Geometry: final body of the model. Coordinates: model frame, mm. A direction names the side the tool comes from. Coordinates: 2 decimals unless noted, no trailing zeros. Loops run counter-clockwise (first coordinate to the right, second up) from the corner with the lowest first, then second, coordinate; pieces in that order, holes last. Notation, with made-up numbers: (72, -40) - (120, -40) arc R17 cw to (120, -16) - close; hole circle Ø6 at (-32, -27). An arc over 180 degrees is marked (long way). Return JSON: item names as keys, results as strings.
from build123d import *

# Parameters (mm, degrees)
SKETCH1_R           = 8
BOSS_EXTRUDE1_DEPTH = 90
SKETCH2_R           = 10
BOSS_EXTRUDE2_DEPTH = 10
BOSS_EXTRUDE3_START = 10
SKETCH3_R           = 10
BOSS_EXTRUDE3_DEPTH = 10
SKETCH4_R           = 7.5
BOSS_EXTRUDE4_DEPTH = 15
BOSS_EXTRUDE5_START = 16
SKETCH5_R           = 7.5
BOSS_EXTRUDE5_DEPTH = 16
SKETCH6_R           = 2.5
CUT_EXTRUDE1_DEPTH  = 16
SKETCH7_R           = 4.5
CUT_EXTRUDE2_DEPTH  = 4
CUT_EXTRUDE3_DEPTH  = 16
SKETCH9_R           = 3
CUT_EXTRUDE4_DEPTH  = 117.53754762


with BuildPart() as part:
    # Sketch1 → Boss-Extrude1 (new body)
    with BuildSketch(Plane.XY):
        with Locations(Location((0, 0, 0), (0, 0, 180))):
            Circle(SKETCH1_R)
    extrude(amount=BOSS_EXTRUDE1_DEPTH)

    # Sketch2 → Boss-Extrude2 (add)
    with BuildSketch(Plane(origin=(0, 0, 0), x_dir=(-1, 0, 0), z_dir=(0, 0, -1))):
        Circle(SKETCH2_R)
    extrude(amount=BOSS_EXTRUDE2_DEPTH)

    # Sketch3 → Boss-Extrude3 (add)
    with BuildSketch(Plane.XY.offset(90).offset(BOSS_EXTRUDE3_START)):
        with Locations(Location((0, 0, 0), (0, 0, 180))):
            Circle(SKETCH3_R)
    extrude(amount=-BOSS_EXTRUDE3_DEPTH)

    # Sketch4 → Boss-Extrude4 (add)
    with BuildSketch(Plane.XY.offset(100)):
        Circle(SKETCH4_R)
    extrude(amount=BOSS_EXTRUDE4_DEPTH)

    # Sketch5 → Boss-Extrude5 (add)
    with BuildSketch(Plane(origin=(0, 0, -10), x_dir=(-1, 0, 0), z_dir=(0, 0, -1)).offset(BOSS_EXTRUDE5_START)):
        with Locations(Location((0, 0, 0), (0, 0, 180))):
            Circle(SKETCH5_R)
    extrude(amount=-BOSS_EXTRUDE5_DEPTH)

    # Sketch6 → Cut-Extrude1 (cut)
    with BuildSketch(Plane.XY.offset(115)):
        Circle(SKETCH6_R)
    extrude(amount=-CUT_EXTRUDE1_DEPTH, mode=Mode.SUBTRACT)

    # Sketch7 → Cut-Extrude2 (cut)
    with BuildSketch(Plane(origin=(0, 10, 0), x_dir=(-1, 0, 0), z_dir=(0, 1, 0))):
        with Locations(Location((0, 95, 0), (0, 0, 90))):
            Circle(SKETCH7_R)
        with Locations(Location((0, -5, 0), (0, 0, 90))):
            Circle(SKETCH7_R)
    extrude(amount=-CUT_EXTRUDE2_DEPTH, mode=Mode.SUBTRACT)

    # Sketch8 → Cut-Extrude3 (cut)
    with BuildSketch(Plane(origin=(0, 0, -26), x_dir=(-1, 0, 0), z_dir=(0, 0, -1))):
        with BuildLine():
            Line((-6, 4.5), (-6, -4.5))
            ThreePointArc((-6, -4.5), (-7.5, 0), (-6, 4.5))
        make_face()
        with BuildLine():
            Line((6, 4.5), (6, -4.5))
            ThreePointArc((6, -4.5), (7.5, 0), (6, 4.5))
        make_face()
    extrude(amount=-CUT_EXTRUDE3_DEPTH, mode=Mode.SUBTRACT)

    # Sketch9 → Cut-Extrude4 (cut, through all)
    with BuildSketch(Plane(origin=(6, 0, 0), x_dir=(0, 0, -1), z_dir=(1, 0, 0))):
        with Locations((19, 0)):
            Circle(SKETCH9_R)
    extrude(amount=-CUT_EXTRUDE4_DEPTH, mode=Mode.SUBTRACT)


solid = part.part
Item 1: Ray query, probe 1 along Z at (x, y) = (0, 7.6); probe 2 along Z at (x, y) = (0.75, -8); probe 3 along X at (y, z) = (-6, 106.5). Return the intervals inside material, ascending. Write a range as from..to.
Worked out:
{"probe 1": "-10..-9.5, -0.5..90.5, 99.5..100", "probe 2": "-10..0, 90..100", "probe 3": "-4.5..4.5"}
Item 2: Mould query, pull axis Z, two halves, no side actions, for faces 1 (the face through (0, 0, 99)), 2 (the face through (0.1, -7.5, -18.1)), 3 (the face through (1.352, 7.584, -0.708)). Classes: +Z half, -Z half, draft (parallel to the pull), parting line (faces both ways), or undercut.
Worked out:
{"face 1": "+Z half", "face 2": "draft", "face 3": "undercut"}
Item 3: Reachability of faces 4 (the face through (-7, 0, -10)), 5 (the face through (-7.493, 0.33, 107.395)), 6 (the face through (-0.1, 7.5, -18.1)), 7 (the face through (-6, 2, -16)), 8 (the face through (6, 2, -16)) from +Z, -Z, +X, -X, +Y, -Y: full face, straight path, thin tool, end or side. Return the list, or none.
Worked out:
{"face 4": "-Z", "face 5": "+Z", "face 6": "-Z, +Y", "face 7": "-Z, -X, +Y, -Y", "face 8": "-Z, +X, +Y, -Y"}
Item 4: Section query D-D, the plane z = 31. Return loops of the section in (x, y), and give its area (3 significant figures).
Worked out:
{"outline": "circle Ø16 at (0, 0)", "area": "201 mm^2"}
Item 5: Section query A-A, the plane y = 0. Return loops of the section in (x, z), and give its area (4 significant figures).
Worked out:
{"outline": "(-10, -10) - (-6, -10) - (-6, -16) - (6, -16) - (6, -10) - (10, -10) - (10, 0) - (8, 0) - (8, 90) - (10, 90) - (10, 100) - (7.5, 100) - (7.5, 115) - (2.5, 115) - (2.5, 99) - (-2.5, 99) - (-2.5, 115) - (-7.5, 115) - (-7.5, 100) - (-10, 100) - (-10, 90) - (-8, 90) - (-8, 0) - (-10, 0) - close; (-6, -26) - (6, -26) - (6, -22) - (-6, -22) - close", "area": "2,105 mm^2"}
Item 6: Section query B-B, the plane z = -19. Return loops of the section in (x, y).
Worked out:
{"outline": "(-6, -4.5) arc R7.5 ccw to (6, -4.5) - (6, -3) - (-6, -3) - close; (-6, 3) - (6, 3) - (6, 4.5) arc R7.5 ccw to (-6, 4.5) - close"}
Item 7: First-contact query: pin 1 Ø3 at (x, z) = (-5.5, 37) entering from -Y; pin 2 Ø8 at (y, z) = (8, 87.5) entering from +X; pin 3 Ø1 at (x, z) = (-7, 31) entering from +Y. Flat tips, straight axial feed; report the tip coordinate or a pass-through.
Worked out:
{"pin 1": "y = -6.93", "pin 2": "x = 8.73", "pin 3": "y = 4.66"}
